The figure shows three views and two pictorial views of one solid part (mm, origin at its lowest corner). Answer the questions. A direction names the side the tool comes from. Coordinates: 2 decimals unless noted, no trailing zeros. Loops run counter-clockwise (first coordinate to the right, second up) from the corner with the lowest first, then second, coordinate; pieces in that order, holes last. Notation, with made-up numbers: (82, -4.5) -> (132, -4.5) arc R28 ccw to (132, 28.5) -> close; hole circle Ø10 at (68.5, 27.25). An arc over 180 degrees is marked (long way). Answer in a Markdown table with one row per item.
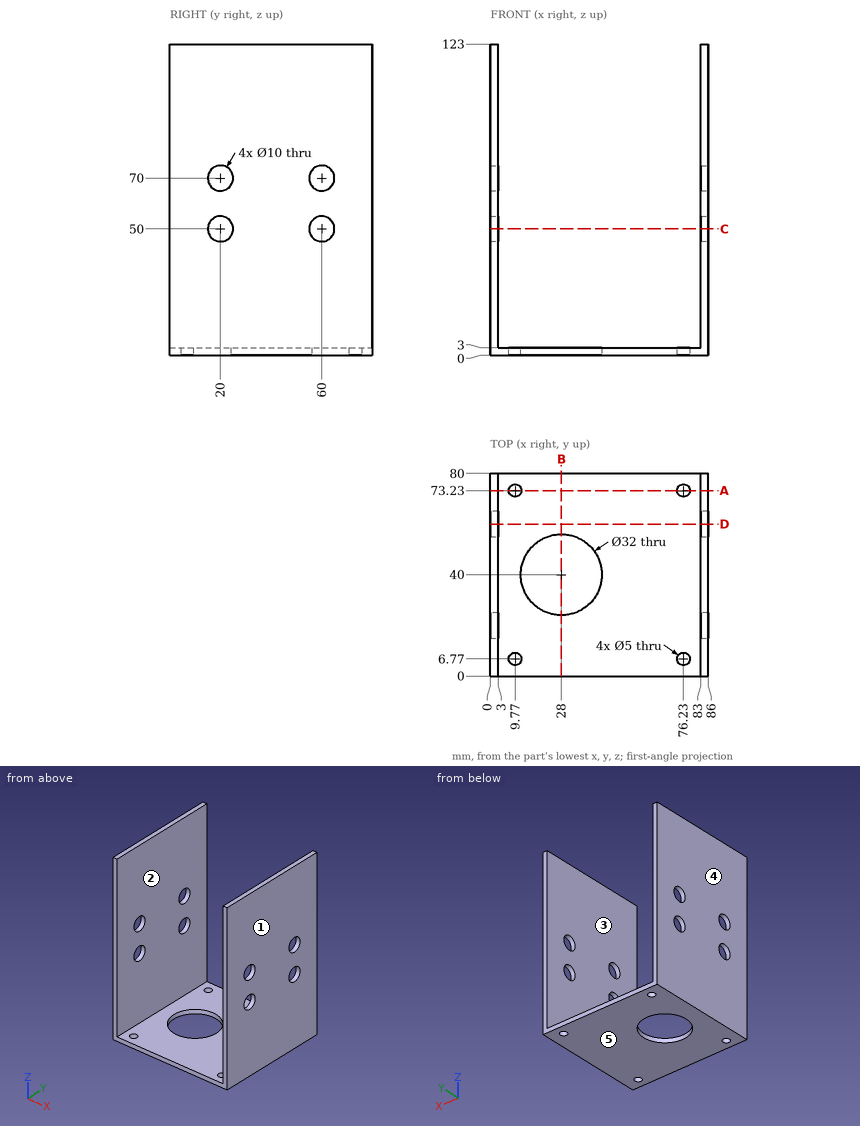
Item 1: A cutting plane is placed at A-A, the plane y = 73.23. Determine the outline of the cut face in (x, z), plus the area to 3 significant figures.
Findings below:
| item | result |
|---|---|
| outline | (0, 0) -> (7.27, 0) -> (7.27, 3) -> (3, 3) -> (3, 123) -> (0, 123) -> close; (12.27, 0) -> (73.73, 0) -> (73.73, 3) -> (12.27, 3) -> close; (78.73, 0) -> (86, 0) -> (86, 123) -> (83, 123) -> (83, 3) -> (78.73, 3) -> close |
| area | 948 mm2 |
Item 2: A cutting plane is placed at B-B, the plane x = 28. Determine the outline of the cut face in (y, z), plus the area to 3 significant figures.
Findings below:
| item | result |
|---|---|
| outline | (0, 0) -> (24, 0) -> (24, 3) -> (0, 3) -> close; (56, 0) -> (80, 0) -> (80, 3) -> (56, 3) -> close |
| area | 144 mm2 |
Item 3: A cutting plane is placed at D-D, the plane y = 60. Determine the outline of the cut face in (x, z), plus the area to 3 significant figures.
Findings below:
| item | result |
|---|---|
| outline | (0, 0) -> (86, 0) -> (86, 45) -> (83, 45) -> (83, 3) -> (3, 3) -> (3, 45) -> (0, 45) -> close; (0, 55) -> (3, 55) -> (3, 65) -> (0, 65) -> close; (0, 75) -> (3, 75) -> (3, 123) -> (0, 123) -> close; (83, 55) -> (86, 55) -> (86, 65) -> (83, 65) -> close; (83, 75) -> (86, 75) -> (86, 123) -> (83, 123) -> close |
| area | 858 mm2 |
Item 4: A tool of negligible diameter and unlimited length cuts with its end or side. For the marked faces 1 and 2, from which of +Z, -Z, +X, -X, +Y, -Y can it reach the whole face along a straight path? Write none if from no direction.
Findings below:
| item | result |
|---|---|
| face 1 | +Z, -Z, +X, +Y, -Y |
| face 2 | +Z, +Y, -Y |
Item 5: A flat-ended cylindrical pin translates along its axis: pin 1 Ø1.5 at (x, y) = (12.5, 51.5) entering from +Z. Find the tip coordinate at first contact, or state that the pin passes through.
Findings below:
| item | result |
|---|---|
| pin 1 | stops at z = 3 |
Item 6: Find the intervals of material crossed by probe 1 along X at (y, z) = (73.23, 0.7); probe 2 along Y at (x, z) = (76, 1); probe 3 along Z at (x, y) = (83.6, 60), in increasing order.
Findings below:
| item | result |
|---|---|
| probe 1 | x = 0 to 7.27, 12.27 to 73.73, 78.73 to 86 |
| probe 2 | y = 0 to 4.28, 9.26 to 70.74, 75.72 to 80 |
| probe 3 | z = 0 to 45, 55 to 65, 75 to 123 |
Item 7: A cutting plane is placed at C-C, the plane z = 50. Determine the outline of the cut face in (x, y), plus the area to 3 significant figures.
Findings below:
| item | result |
|---|---|
| outline | (0, 0) -> (3, 0) -> (3, 15) -> (0, 15) -> close; (0, 25) -> (3, 25) -> (3, 55) -> (0, 55) -> close; (0, 65) -> (3, 65) -> (3, 80) -> (0, 80) -> close; (83, 0) -> (86, 0) -> (86, 15) -> (83, 15) -> close; (83, 25) -> (86, 25) -> (86, 55) -> (83, 55) -> close; (83, 65) -> (86, 65) -> (86, 80) -> (83, 80) -> close |
| area | 360 mm2 |
Item 8: Determine the mould class of the marked faces 3, 4 and 5 for opening direction X: +X half, -X half, draft (parallel to the pull), parting line (faces both ways), or undercut.
Findings below:
| item | result |
|---|---|
| face 3 | undercut |
| face 4 | -X half |
| face 5 | draft |
